```python
from build123d import *

# Parameters (mm, degrees)
SKETCH_W              = 76
SKETCH_H              = 37
PAD_DEPTH             = 30
SKETCH020_R           = 14
POCKET_DEPTH          = 8
SKETCH026_R           = 1.7
PAD001_DEPTH          = 2
POCKET001_DEPTH       = 5
POLARPATTERN_COUNT    = 6
SKETCH025_R           = 1.7
POCKET005_DEPTH       = 212.317184
POLARPATTERN001_COUNT = 6
SKETCH022_R           = 1.7
SKETCH022_R_2         = 7
SKETCH022_W           = 3.5
SKETCH022_H           = 5
POCKET002_DEPTH       = 5
SKETCH027_W           = 5
SKETCH027_H           = 30
POCKET006_DEPTH       = 5.001
SKETCH028_R           = 1.6
POCKET007_DEPTH       = 5
POCKET008_DEPTH       = 2
FILLET_R              = 7
FILLET001_R           = 7
FILLET002_R           = 5
FILLET003_R           = 5
FILLET004_R           = 3
FILLET005_R           = 3
FILLET006_R           = 3
FILLET007_R           = 3
FILLET008_R           = 2
FILLET009_R           = 2


with BuildPart() as part:
    # Sketch → Pad (new body, symmetric)
    with BuildSketch(Plane.XY):
        Rectangle(SKETCH_W, SKETCH_H)
        Polygon((-34, -11.5), (-30, -15.5), (30, -15.5), (34, -11.5), (34, 12.5), (12.5, 13.5), (-12.5, 13.5), (-34, 12.5), align=None, mode=Mode.SUBTRACT)
    extrude(amount=PAD_DEPTH, both=True)

    # Sketch020 → Pocket (cut)
    with BuildSketch(Plane(origin=(0, 18.5, 0), x_dir=(-1, 0, 0), z_dir=(0, 1, 0))):
        Circle(SKETCH020_R)
    extrude(amount=-POCKET_DEPTH, mode=Mode.SUBTRACT)

    # Sketch026 → Pad001 (new body)
    with BuildSketch(Plane.XZ.offset(-13.5)):
        with Locations((20, 0)):
            Circle(SKETCH026_R)
    extrude(amount=PAD001_DEPTH)

    # Sketch021 → Pocket001 (cut)
    with BuildSketch(Plane.XZ.offset(-11.5)):
        Polygon((18.383419, 2.8), (16.766838, 0), (18.383419, -2.8), (21.616581, -2.8), (23.233162, 0), (21.616581, 2.8), align=None)
    pocket001 = extrude(amount=-POCKET001_DEPTH, mode=Mode.SUBTRACT)

    # PolarPattern: Pocket001 ×6 about axis
    polarpattern_axis = Axis((0, 11.5, 0), (0, -1, 0))
    for i in range(1, POLARPATTERN_COUNT):
        add(pocket001.rotate(polarpattern_axis, i * 360 / POLARPATTERN_COUNT), mode=Mode.SUBTRACT)

    # Sketch025 → Pocket005 (cut, through all)
    with BuildSketch(Plane.XZ.offset(-13.5)):
        with Locations((20, 0)):
            Circle(SKETCH025_R)
    pocket005 = extrude(amount=-POCKET005_DEPTH, mode=Mode.SUBTRACT)

    # PolarPattern001: Pocket005 ×6 about axis
    polarpattern001_axis = Axis((0, 13.5, 0), (0, -1, 0))
    for i in range(1, POLARPATTERN001_COUNT):
        add(pocket005.rotate(polarpattern001_axis, i * 360 / POLARPATTERN001_COUNT), mode=Mode.SUBTRACT)

    # Sketch022 → Pocket002 (cut)
    with BuildSketch(Plane.XZ.offset(18.5)):
        with Locations((0, 22)):
            Circle(SKETCH022_R)
        with Locations((0, -22)):
            Circle(SKETCH022_R)
        with Locations((-22, 0)):
            Circle(SKETCH022_R)
        with Locations((22, 0)):
            Circle(SKETCH022_R)
        Circle(SKETCH022_R_2)
        with Locations((-15, 0)):
            Circle(SKETCH022_R)
        with BuildLine():
            ThreePointArc((-23.660997, 14.014536), (-21.731705, 6.47943), (-14.196598, 8.408722))
            ThreePointArc((-8.408722, 14.196598), (-11.667262, 11.667262), (-14.196598, 8.408722))
            ThreePointArc((-8.408722, 14.196598), (-6.47943, 21.731705), (-14.014536, 23.660997))
            ThreePointArc((-14.014536, 23.660997), (-19.445436, 19.445436), (-23.660997, 14.014536))
        make_face()
        with BuildLine():
            ThreePointArc((8.408722, -14.196598), (11.667262, -11.667262), (14.196598, -8.408722))
            ThreePointArc((23.660997, -14.014536), (21.731705, -6.47943), (14.196598, -8.408722))
            ThreePointArc((14.014536, -23.660997), (19.445436, -19.445436), (23.660997, -14.014536))
            ThreePointArc((8.408722, -14.196598), (6.47943, -21.731705), (14.014536, -23.660997))
        make_face()
        with BuildLine():
            ThreePointArc((23.660997, 14.014536), (19.445436, 19.445436), (14.014536, 23.660997))
            ThreePointArc((14.014536, 23.660997), (6.47943, 21.731705), (8.408722, 14.196598))
            ThreePointArc((14.196598, 8.408722), (11.667262, 11.667262), (8.408722, 14.196598))
            ThreePointArc((14.196598, 8.408722), (21.731705, 6.47943), (23.660997, 14.014536))
        make_face()
        with BuildLine():
            ThreePointArc((-14.014536, -23.660997), (-6.47943, -21.731705), (-8.408722, -14.196598))
            ThreePointArc((-14.196598, -8.408722), (-11.667262, -11.667262), (-8.408722, -14.196598))
            ThreePointArc((-14.196598, -8.408722), (-21.731705, -6.47943), (-23.660997, -14.014536))
            ThreePointArc((-23.660997, -14.014536), (-19.445436, -19.445436), (-14.014536, -23.660997))
        make_face()
        with Locations((-10.25, 0)):
            Rectangle(SKETCH022_W, SKETCH022_H)
    extrude(amount=-POCKET002_DEPTH, mode=Mode.SUBTRACT)

    # Sketch027 → Pocket006 (cut, through all)
    with BuildSketch(Plane.XZ.offset(-13.5)):
        with Locations((0, 15)):
            Rectangle(SKETCH027_W, SKETCH027_H)
    extrude(amount=-POCKET006_DEPTH, mode=Mode.SUBTRACT)

    # Sketch028 → Pocket007 (cut)
    with BuildSketch(Plane(origin=(-38, 0, 0), x_dir=(0, -1, 0), z_dir=(-1, 0, 0))):
        with Locations((4, 22.5)):
            Circle(SKETCH028_R)
        with Locations((4, -22.5)):
            Circle(SKETCH028_R)
        with BuildLine():
            ThreePointArc((11, 10), (4, 17), (-3, 10))
            Line((-3, 10), (-3, -10))
            ThreePointArc((-3, -10), (4, -17), (11, -10))
            Line((11, 10), (11, -10))
        make_face()
    extrude(amount=-POCKET007_DEPTH, mode=Mode.SUBTRACT)

    # Sketch029 → Pocket008 (cut)
    with BuildSketch(Plane.YZ.offset(-34)):
        Polygon((-2.383419, 19.7), (-0.766838, 22.5), (-2.383419, 25.3), (-5.616581, 25.3), (-7.233162, 22.5), (-5.616581, 19.7), align=None)
        Polygon((-7.233162, -22.5), (-5.616581, -25.3), (-2.383419, -25.3), (-0.766838, -22.5), (-2.383419, -19.7), (-5.616581, -19.7), align=None)
    extrude(amount=-POCKET008_DEPTH, mode=Mode.SUBTRACT)

    # Fillet
    fillet_edges = [part.edges().sort_by_distance(p)[0] for p in [
        (-38, -18.5, 0),
    ]]
    fillet(fillet_edges, radius=FILLET_R)

    # Fillet001
    fillet001_edges = [part.edges().sort_by_distance(p)[0] for p in [
        (38, -18.5, 0),
    ]]
    fillet(fillet001_edges, radius=FILLET001_R)

    # Fillet002
    fillet002_edges = [part.edges().sort_by_distance(p)[0] for p in [
        (-34, 12.5, 0),
    ]]
    fillet(fillet002_edges, radius=FILLET002_R)

    # Fillet003
    fillet003_edges = [part.edges().sort_by_distance(p)[0] for p in [
        (34, 12.5, 0),
    ]]
    fillet(fillet003_edges, radius=FILLET003_R)

    # Fillet004
    fillet004_edges = [part.edges().sort_by_distance(p)[0] for p in [
        (-30, -15.5, 0),
    ]]
    fillet(fillet004_edges, radius=FILLET004_R)

    # Fillet005
    fillet005_edges = [part.edges().sort_by_distance(p)[0] for p in [
        (30, -15.5, 0),
    ]]
    fillet(fillet005_edges, radius=FILLET005_R)

    # Fillet006
    fillet006_edges = [part.edges().sort_by_distance(p)[0] for p in [
        (34, -11.5, 0),
    ]]
    fillet(fillet006_edges, radius=FILLET006_R)

    # Fillet007
    fillet007_edges = [part.edges().sort_by_distance(p)[0] for p in [
        (-34, -11.5, 0),
    ]]
    fillet(fillet007_edges, radius=FILLET007_R)

    # Fillet008
    fillet008_edges = [part.edges().sort_by_distance(p)[0] for p in [
        (-2.5, 16, 13.774977),
    ]]
    fillet(fillet008_edges, radius=FILLET008_R)

    # Fillet009
    fillet009_edges = [part.edges().sort_by_distance(p)[0] for p in [
        (2.5, 16, 13.774977),
    ]]
    fillet(fillet009_edges, radius=FILLET009_R)


solid = part.part
```
Here's how the part is built. I have some questions about the finished solid (model axes, mm). A direction names the side the tool comes from. Round coordinates to 2 decimals unless told otherwise and drop trailing zeros. Order: outer loops, then holes, each group sorted by start corner. A loop starts at its lowest first (then second) coordinate and runs counter-clockwise, first axis right, second up. Notation, with made-up numbers: (76, -10.5) -> (121, -10.5) arc R34 ccw to (121, 26.5) -> close; hole circle Ø2 at (-34, 74). An arc over 180 degrees is marked (long way). Use a Markdown table: item, result. Add a question column.
(1) For pin 1 Ø4.5 at (x, z) = (10, 17.32) entering from +Y; pin 2 Ø4 at (y, z) = (-14.5, -1) entering from +X; pin 3 Ø4.5 at (x, z) = (-10, -17.32) entering from -Y, each with a flat end and sliding along its axis, tell me the tip position at first contact or that it passes through.
(2) Suppose I cut it at A-A, the plane x = 0. Please give me the cut outline in (y, z).
(3) Suppose I cut it at B-B, the plane x = 10. Count the separate pieces of the cut face and the enclosed holes in it, and give its area (3 significant figures).
(4) I need wall thicknesses on line 1 along Z through (x, y) = (0, -17); line 2 along X through (y, z) = (-7, 20.5); line 3 along Y through (x, z) = (11.5, -26). Which ranges of each line are inside material? Lowest first, please.
(5) For faces 1 (the face through (-19.51, -17.02, -19.38)), 2 (the face through (-34.986, -6.414, 23.92)), 3 (the face through (-33.765, -11.421, 21.687)), which set-ups out of +Z, -Z, +X, -X, +Y, -Y let a thin tool reach every point of the face, with its end or its side?
(6) If we mould it in two halves opening along Z, with no side actions, what happens to faces 4 (the face through (-36, -3, -21)), 5 (the face through (-34, 5, 0)), 6 (the face through (-20.43, -17.02, -0.65))? For each: released by +Z, released by -Z, zero draft, split by the parting line, or undercut.
Verdict:
| question | item | result |
|---|---|---|
| 1 | pin 1 | y = 18.5 |
| 1 | pin 2 | x = 37.93 |
| 1 | pin 3 | y = 16.5 |
| 2 | outline | (-18.5, -30) -> (-15.5, -30) -> (-15.5, -23.7) -> (-18.5, -23.7) -> close; (-18.5, -20.3) -> (-15.5, -20.3) -> (-15.5, -7) -> (-18.5, -7) -> close; (-18.5, 7) -> (-15.5, 7) -> (-15.5, 20.3) -> (-18.5, 20.3) -> close; (-18.5, 23.7) -> (-15.5, 23.7) -> (-15.5, 30) -> (-18.5, 30) -> close; (13.5, -30) -> (18.5, -30) -> (18.5, -14) -> (13.5, -14) -> close |
| 3 | separate pieces | 7 |
| 3 | enclosed holes | 0 |
| 3 | area | 268 mm2 |
| 4 | line 1 | -30 to -23.7, -20.3 to -7, 7 to 20.3, 23.7 to 30 |
| 4 | line 2 | -38 to -34, 34 to 38 |
| 4 | line 3 | -18.5 to -15.5, 13.5 to 18.5 |
| 5 | face 1 | -Y |
| 5 | face 2 | none |
| 5 | face 3 | +Z, -Z |
| 6 | face 4 | undercut |
| 6 | face 5 | zero draft |
| 6 | face 6 | undercut |
